Autodesk Inventor part; units mm, degrees
ref_plane "YZ Plane" through (0, 0, 0) normal (1, 0, 0) x (0, 1, 0)
ref_plane "XZ Plane" through (0, 0, 0) normal (0, 1, 0) x (-1, 0, 0)
ref_plane "XY Plane" through (0, 0, 0) normal (0, 0, 1) x (1, 0, 0)
sketch "Sketch1" plane through (0, 0, 0) normal (1, 0, 0) x (0, 1, 0)
  line L0 (0, 0) -> (66, 0)
  line L1 (66, 0) -> (66, 91.5)
  line L2 (66, 91.5) -> (0, 91.5)
  line L3 (0, 91.5) -> (0, 0)
  dimension "d0" = 91.5
  dimension "d1" = 66
extrude "Extrusion1" add sketch "Sketch1" along normal blind 5
fillet "Fillet1" radius 1 4 edges at (2.5, 0, 91.5) (2.5, 0, 0) (2.5, 66, 0) (2.5, 66, 91.5)
sketch "Sketch2" plane through (5, 0, 0) normal (1, 0, 0) x (0, 0, -1)
  line L0 (-86.5, 5) -> (-5, 5)
  line L1 (-5, 5) -> (-5, 61)
  line L2 (-5, 61) -> (-86.5, 61)
  line L3 (-86.5, 61) -> (-86.5, 5)
  line L4 (-90.5, 0) -> (-1, 0)
  line L5 (0, 1) -> (0, 65)
  line L6 (-1, 66) -> (-90.5, 66)
  line L7 (-91.5, 65) -> (-91.5, 1)
  point P0 (0, 0)
  dimension "d5" = 5
  dimension "d6" = 5
  dimension "d7" = 5
  dimension "d8" = 5
extrude "Extrusion2" add sketch "Sketch2" along normal blind 3
chamfer "Chamfer1" distance 2 angle 45 4 edges at (6.5, 61, 86.5) (6.5, 5, 86.5) (6.5, 5, 5) (6.5, 61, 5)
sketch "Sketch3" plane through (8, 0, 0) normal (1, 0, 0) x (0, 0, -1)
  line L0 (-81.5, 56) -> (-10, 56)
  line L1 (-10, 56) -> (-10, 10)
  line L2 (-10, 10) -> (-81.5, 10)
  line L3 (-81.5, 10) -> (-81.5, 56)
  line L4 (-5, 7) -> (-5, 59)
  line L5 (-7, 61) -> (-84.5, 61)
  line L6 (-86.5, 59) -> (-86.5, 7)
  line L7 (-84.5, 5) -> (-7, 5)
  point P0 (0, 0)
  dimension "d14" = 5
  dimension "d15" = 5
  dimension "d17" = 5
  dimension "d18" = 5
extrude "Extrusion3" cut sketch "Sketch3" against normal blind 3
chamfer "Chamfer2" distance 2 angle 45 4 edges at (6.5, 56, 81.5) (6.5, 56, 10) (6.5, 10, 81.5) (6.5, 10, 10)
sketch "Sketch4" plane through (0, 0, 0) normal (-1, 0, 0) x (0, 0, 1)
  line L0 (3, 3) -> (88.5, 3)
  line L1 (88.5, 3) -> (88.5, 63)
  line L2 (88.5, 63) -> (3, 63)
  line L3 (3, 63) -> (3, 3)
  line L4 (90.5, 0) -> (1, 0)
  line L5 (91.5, 65) -> (91.5, 1)
  line L6 (1, 66) -> (90.5, 66)
  line L7 (0, 1) -> (0, 65)
  point P0 (0, 0)
  dimension "d24" = 3
  dimension "d25" = 3
  dimension "d26" = 3
  dimension "d27" = 3
hole "Hole1" at (0, 63, 88.5) at (0, 3, 88.5) at (0, 3, 3) at (0, 63, 3) direction (1, 0, 0) diameter 3.3 end through all
properties part number "couverclePCB"
Build history of the part. All positions in model axes, mm. A direction names the side the tool comes from. Coordinates: 2 decimals unless noted, no trailing zeros. Order: outer loops, then holes, each group sorted by start corner. A loop starts at its lowest first (then second) coordinate and runs counter-clockwise, first axis right, second up. Notation, with made-up numbers: M 47,19.25 L 98,19.25 A20 cw 98,58.25 Z; hole C -13.5,67 d10. An arc over 180 degrees is marked long. One line per question, with ' | ' between items. Start each with the question number.
1. Wall check: line 1 along Z through (x, y) = (2.1, 3); line 2 along Y through (x, z) = (1.2, 3); line 3 along Y through (x, z) = (7, 39.5). Give the ranges that are in metal, low to high. Write a range as [from, to].
2. Cut at C-C (x = 6). Write the cut outline in (y, z), plus the area to 4 significant figures.
3. Mould opens along Y. For faces 5 (the face through (6, 33, 86.5)), 6 (the face through (7, 33, 10)), 7 (the face through (6, 61, 45)) say: +Y half, -Y half, draft (parallel to the pull), parting line (faces both ways), or undercut.
4. Cut at B-B (z = 88.5). Write the cut outline in (x, y).
5. Tool access for faces 1 (the face through (6.5, 60, 85.5)), 2 (the face through (7, 6, 6)), 3 (the face through (7, 33, 81.5)), 4 (the face through (7, 60, 6)): list every direction of +Z, -Z, +X, -X, +Y, -Y with a clear straight run to the whole face (end or side of a thin tool).
6. Flat gauge pins, fed straight in: P1, Ø2.5, axis at x = 7, y = 42, coming from the +Z side; P2, Ø1.5, axis at y = 52, z = 56.5, coming from the +X side; P3, Ø1.5, axis at x = 7, z = 79.5, coming from the +Y side. Where does each tip first touch, or does it go through?
7. Cut at D-D (y = 8.5). Write the cut outline in (x, z).
8. Cut at A-A (y = 63). Write the cut outline in (x, z).
The answers:
1) line 1: z = [0, 1.35], [4.65, 86.85], [90.15, 91.5] | line 2: y = [0, 1.35], [4.65, 61.35], [64.65, 66] | line 3: y = [5, 10], [56, 61]
2) outline: M 5,7 L 7,5 L 59,5 L 61,7 L 61,84.5 L 59,86.5 L 7,86.5 L 5,84.5 Z; hole M 10,12 L 12,10 L 54,10 L 56,12 L 56,79.5 L 54,81.5 L 12,81.5 L 10,79.5 Z | area: 1,275 mm2
3) face 5: draft | face 6: undercut | face 7: +Y half
4) outline: M 0,0 L 5,0 L 5,1.35 L 0,1.35 Z; M 0,4.65 L 5,4.65 L 5,61.35 L 0,61.35 Z; M 0,64.65 L 5,64.65 L 5,66 L 0,66 Z
5) face 1: +Z, +X, +Y | face 2: -Z, +X, -Y | face 3: +X | face 4: -Z, +X, +Y
6) P1: stops at z = 86.5 | P2: stops at x = 5 | P3: stops at y = 61
7) outline: M 0,0 L 5,0 L 5,5 L 8,5 L 8,86.5 L 5,86.5 L 5,91.5 L 0,91.5 Z
8) outline: M 0,0 L 5,0 L 5,1.35 L 0,1.35 Z; M 0,4.65 L 5,4.65 L 5,86.85 L 0,86.85 Z; M 0,90.15 L 5,90.15 L 5,91.5 L 0,91.5 Z
